Could you check a few things on this drawing? It's one solid part, dimensions in mm from its lowest x, y, z. Coordinates: 2 decimals unless noted, no trailing zeros. Order: outer loops, then holes, each group sorted by start corner. A loop starts at its lowest first (then second) coordinate and runs counter-clockwise, first axis right, second up. Notation, with made-up numbers: (26.25, 18.25) - (70.25, 18.25) arc R17 ccw to (70.25, 23.25) - close; hole circle Ø11 at (52, -38). An arc over 180 degrees is marked (long way). Answer in a Markdown table with one row per item. Add a question column.
Item 1: Will these pins go through, and if not, where does the flat tip stop? pin 1 Ø3.5 at (x, z) = (86, 45) entering from +Y (1 decimal); pin 2 Ø4.5 at (x, z) = (82.55, 12.7) entering from -Y; pin 3 Ø1 at (x, y) = (48.5, 4.5) entering from -Z.
Item 2: I want a section at A-A (z = 44.45). Count the separate pieces of the cut face and the enclosed holes in it.
Item 3: Thinking about a two-plate mould opening in X: for the marked faces 1 and 2, which applies, +X half, -X half, draft (parallel to the pull), parting line (faces both ways), or undercut?
Item 4: I want a section at B-B (x = 82.55). Please give me the cut outline in (y, z).
Item 5: I want a section at C-C (z = 12.7). Please give me the cut outline in (x, y).
Item 6: If I drill on line 1 along X through (y, z) = (1.75, 44.45) (1 decimal); line 2 along Z through (x, y) = (19.05, 4.75); line 3 along X through (y, z) = (3.75, 43.5) (1 decimal), over which ranges is the centre line in solid material (lowest first)? Write a range as from..to.
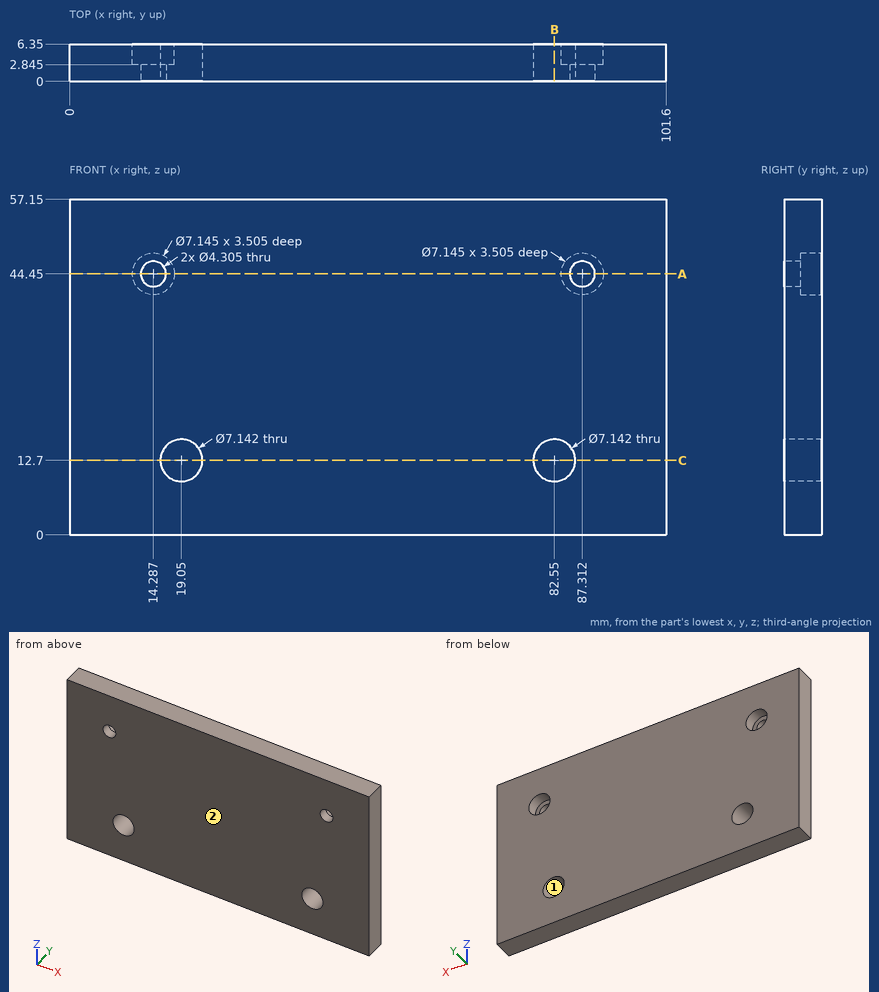
Values follow:
| question | item | result |
|---|---|---|
| 1 | pin 1 | stops at y = 2.8 |
| 1 | pin 2 | passes through |
| 1 | pin 3 | stops at z = 0 |
| 2 | separate pieces | 3 |
| 2 | enclosed holes | 0 |
| 3 | face 1 | undercut |
| 3 | face 2 | draft |
| 4 | outline | (0, 0) - (6.35, 0) - (6.35, 9.13) - (0, 9.13) - close; (0, 16.27) - (6.35, 16.27) - (6.35, 57.15) - (0, 57.15) - close |
| 5 | outline | (0, 0) - (15.48, 0) - (15.48, 6.35) - (0, 6.35) - close; (22.62, 0) - (78.98, 0) - (78.98, 6.35) - (22.62, 6.35) - close; (86.12, 0) - (101.6, 0) - (101.6, 6.35) - (86.12, 6.35) - close |
| 6 | line 1 | x = 0..12.1, 16.4..85.2, 89.5..101.6 |
| 6 | line 2 | z = 0..9.13, 16.27..57.15 |
| 6 | line 3 | x = 0..10.8, 17.7..83.9, 90.8..101.6 |
